Geometry: see drawing. Coordinates: mm, zero at the bounding-box minimum. A direction names the side the tool comes from. Round coordinates to 2 decimals unless told otherwise and drop trailing zeros. Loops run counter-clockwise (first coordinate to the right, second up) from the corner with the lowest first, then second, coordinate; pieces in that order, holes last. Notation, with made-up numbers: (78.5, 30) -> (107.5, 30) arc R20 ccw to (107.5, 40) -> close; hole circle Ø7 at (12.5, -4). An arc over 180 degrees is marked (long way). Answer in a Markdown table with one row per item.
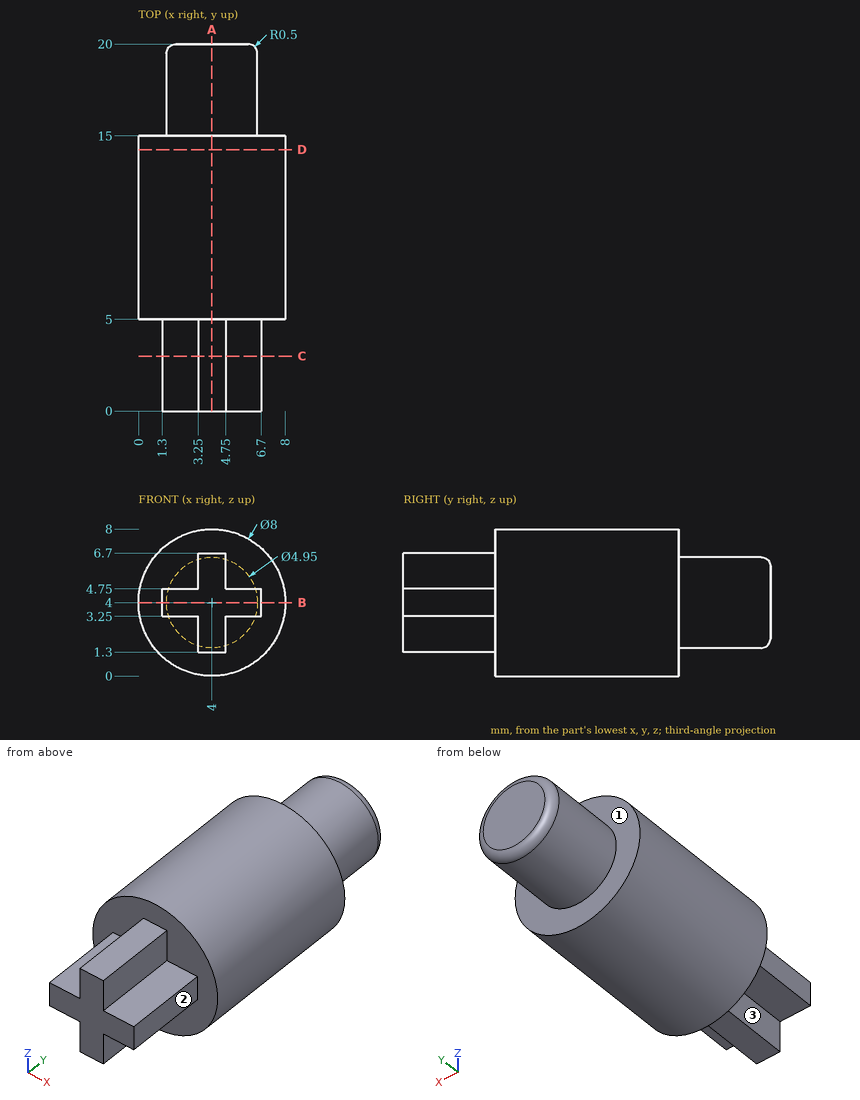
Item 1: Section query B-B, the plane z = 4. Output: boundary loops of the cut face in (x, y) (3 decimals), and give its area (3 significant figures).
Ans:
| item | result |
|---|---|
| outline | (0, 5) -> (1.3, 5) -> (1.3, 0) -> (6.7, 0) -> (6.7, 5) -> (8, 5) -> (8, 15) -> (6.475, 15) -> (6.475, 19.5) arc R0.5 ccw to (5.975, 20) -> (2.025, 20) arc R0.5 ccw to (1.525, 19.5) -> (1.525, 15) -> (0, 15) -> close |
| area | 132 mm2 |
Item 2: First-contact query: P1, Ø2, axis at x = 6, y = 3, coming from the +Z side; P2, Ø1.2, axis at x = 4, y = 3.5, coming from the +Z side; P3, Ø2, axis at y = 3, z = 5.5, coming from the -X side. Flat tips, straight axial feed; report the tip coordinate or a pass-through.
Ans:
| item | result |
|---|---|
| P1 | z = 4.75 |
| P2 | z = 6.7 |
| P3 | x = 1.3 |
Item 3: Section query C-C, the plane y = 3. Output: boundary loops of the cut face in (x, z), and give its area (4 significant figures).
Ans:
| item | result |
|---|---|
| outline | (1.3, 3.25) -> (3.25, 3.25) -> (3.25, 1.3) -> (4.75, 1.3) -> (4.75, 3.25) -> (6.7, 3.25) -> (6.7, 4.75) -> (4.75, 4.75) -> (4.75, 6.7) -> (3.25, 6.7) -> (3.25, 4.75) -> (1.3, 4.75) -> close |
| area | 13.95 mm2 |
Item 4: Ray query, L1, parallel to X at y = 1.75, z = 6.5; L2, parallel to Y at x = 2.25, z = 0.5; L3, parallel to Z at x = 4.25, y = 1. Return the intervals inside material, ascending.
Ans:
| item | result |
|---|---|
| L1 | 3.25 to 4.75 |
| L2 | 5 to 15 |
| L3 | 1.3 to 6.7 |
Item 5: Section query D-D, the plane y = 14.25. Output: boundary loops of the cut face in (x, z), and give its area (3 significant figures).
Ans:
| item | result |
|---|---|
| outline | circle Ø8 at (4, 4) |
| area | 50.3 mm2 |
Item 6: Section query A-A, the plane x = 4. Output: boundary loops of the cut face in (y, z) (3 decimals), and give its area (3 significant figures).
Ans:
| item | result |
|---|---|
| outline | (0, 1.3) -> (5, 1.3) -> (5, 0) -> (15, 0) -> (15, 1.525) -> (19.5, 1.525) arc R0.5 ccw to (20, 2.025) -> (20, 5.975) arc R0.5 ccw to (19.5, 6.475) -> (15, 6.475) -> (15, 8) -> (5, 8) -> (5, 6.7) -> (0, 6.7) -> close |
| area | 132 mm2 |
Item 7: Set-up query: the marked faces 1, 2 and 3. Return all of +Z, -Z, +X, -X, +Y, -Y with unobstructed straight access to the full face (end or side cutting, diameter ignored); none if empty.
Ans:
| item | result |
|---|---|
| face 1 | +Y |
| face 2 | +Z, -Z, +X, -Y |
| face 3 | -Z, -X, -Y |
